The figure shows three views and two pictorial views of one solid part (mm, origin at its lowest corner). Answer the questions. Coordinates: 2 decimals unless noted, no trailing zeros. Order: outer loops, then holes, each group sorted by start corner. A loop starts at its lowest first (then second) coordinate and runs counter-clockwise, first axis right, second up. Notation, with made-up numbers: (42, 48.5) - (83, 48.5) arc R30 ccw to (83, 73.5) - close; hole circle Ø7 at (-29, -14.75). An arc over 180 degrees is marked (long way). Use one line per item in the form item = value. Start each with the question number.
Item 1: Section A-A, the plane y = 0.9 is taken. Write down the section's boundary in (x, z).
Item 2: Consider line 1 along Z through (x, y) = (5, 2.35); line 2 along X through (y, z) = (3.25, 6.5); line 3 along X through (y, z) = (0.85, 5.75). Determine where each line is inside the solid, lowest interval first. Write a range as [from, to].
Item 3: The mould has two halves that part along Z. Classify the marked faces 1, 2 and 3: released by +Z, released by -Z, zero draft, split by the parting line, or undercut.
Item 4: Each of these flat-tipped pins is pushed along its axis until it touches: pin 1 Ø3 at (x, z) = (5, 5) entering from -Y; pin 2 Ø1.5 at (y, z) = (2, 2) entering from +X; pin 3 Ø2 at (x, y) = (7, 1.5) entering from +Z. Where does it stop, or does it pass through?
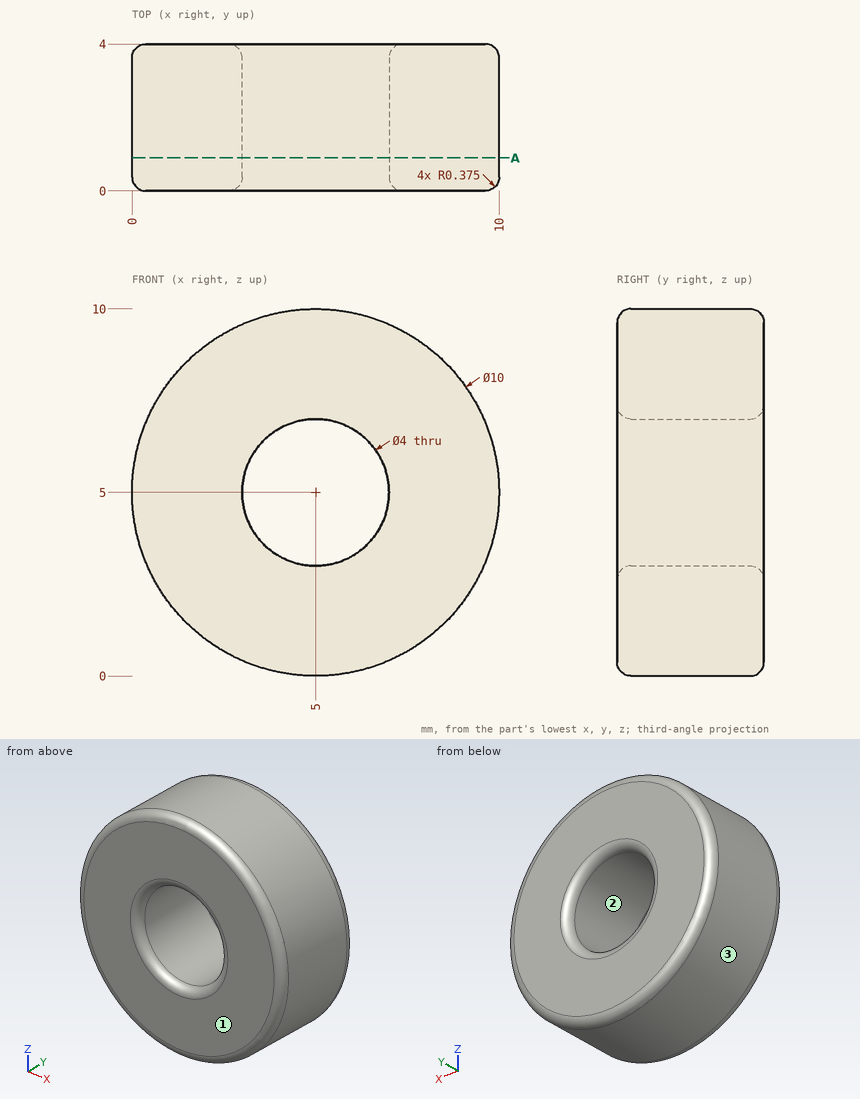
Response:
q1.outline = circle Ø10 at (5, 5); hole circle Ø4 at (5, 5)
q2.line_1 = [0, 3], [7, 10]
q2.line_2 = [0.23, 3.68], [6.32, 9.77]
q2.line_3 = [0.06, 3.15], [6.85, 9.94]
q3.face_1 = zero draft
q3.face_2 = undercut
q3.face_3 = split by the parting line
q4.pin_1 = through
q4.pin_2 = 9.47
q4.pin_3 = 9.9
